Autodesk Inventor part; units mm, degrees
ref_plane "YZ Plane" through (0, 0, 0) normal (1, 0, 0) x (0, 1, 0)
ref_plane "XZ Plane" through (0, 0, 0) normal (0, 1, 0) x (-1, 0, 0)
ref_plane "XY Plane" through (0, 0, 0) normal (0, 0, 1) x (1, 0, 0)
sketch "スケッチ1" plane through (0, 0, 0) normal (0, 0, 1) x (1, 0, 0)
  line L0 (9, 0) -> (9, 4)
  line L1 (9, 12) -> (2.2731, 12)
  line L2 (0, 8) -> (9, 8)
  line L3 (0, 4) -> (9, 4)
  line L4 (9, 8) -> (9, 12)
  line L5 (2.2731, 12) -> (0, 14.2779)
  line L6 (2.2731, 0) -> (-5.7099, -8)
  line L7 (-5.7099, 20) -> (-15.7099, 20)
  line L8 (-5.7099, -8) -> (-15.7099, -8)
  line L9 (-15.7099, 20) -> (-25.7698, 20)
  line L10 (-25.7698, 20) -> (-25.7698, -8)
  line L11 (-25.7698, -8) -> (-15.7099, -8)
  line L12 (2.2731, 0) -> (9, 0)
  line L13 (0, 14.2779) -> (-5.7099, 20)
  arc A0 (-2.1881, 8) -> (-2.1881, 4) centre (-5.7099, 6) ccw
  line L14 (0, 8) -> (-2.1881, 8)
  line L15 (0, 4) -> (-2.1881, 4)
  point P0 (0, 0)
  point P1 (4.5, 12)
  point P2 (4.5, 0)
  point P3 (4.5, 4)
  point P4 (-25.7099, 6)
  dimension "d5" = 4
  dimension "d8" = 10
  dimension "d9" = 10
  dimension "d12" = 14
  dimension "d90" = 8.1
extrude "押し出し1" add sketch "スケッチ1" along normal blind 6
sketch "スケッチ2" plane through (0, 0, 6) normal (0, 0, 1) x (1, 0, 0)
  circle A0 centre (5.6365, 13.3) radius 1.5
  line L0 (9, 8) -> (9, 12)
  line L1 (11.5477, 6) -> (-28.1936, 6) construction
  line L2 (9, 12) -> (2.2731, 12)
  circle A1 centre (5.6365, -1.3) radius 1.5
  point P0 (0, 0)
  point P1 (4.8882, 12)
  point P2 (6.3849, 12)
  dimension "d15" = 3
  dimension "d16" = 3.3635
  dimension "d17" = 1.3
extrude "押し出し2" cut sketch "スケッチ2" against normal blind 6 contours A0 L2 | A1 picked at (5.4614, 13.0013)
sketch "スケッチ3" plane through (0, 0, 6) normal (0, 0, 1) x (1, 0, 0)
  circle A0 centre (5.6365, 13.3) radius 1.5
  line L0 (9, 12) -> (2.2731, 12)
  point P0 (0, 0)
  point P1 (4.8882, 12)
  point P2 (6.3849, 12)
  dimension "d20" = 3
  dimension "d21" = 1.3
extrude "押し出し3" add sketch "スケッチ3" against normal blind 6 contours A0 L0 picked at (5.4614, 13.0013)
sketch "スケッチ4" plane through (0, 0, 6) normal (0, 0, 1) x (1, 0, 0)
  arc A0 (6.3849, 12) -> (4.8882, 12) centre (5.6365, 13.3) ccw
  circle A1 centre (5.6365, 13.3) radius 1.5
  point P0 (0, 0)
  dimension "d24" = 3
extrude "押し出し4" cut sketch "スケッチ4" against normal blind 6
fillet "フィレット1" radius 5 1 edges at (-25.7698, 20, 3)
fillet "フィレット2" radius 5 1 edges at (-25.7698, -8, 3)
fillet "フィレット3" radius 3 4 edges at (-5.7099, -8, 3) (2.2731, 0, 3) (-5.7099, 20, 3) (2.2731, 12, 3)
sketch "スケッチ6" plane through (0, 4, 0) normal (0, 1, 0) x (1, 0, 0)
  point P0 (0, 0)
sketch "スケッチ7" plane through (4.8882, 12, 6) normal (0, 1, 0) x (1, 0, 0)
  circle A0 centre (0.7488, 3) radius 1.6
  line L0 (1.4967, 0) -> (0, 0)
  line L1 (4.1118, 6) -> (4.1118, 0)
  point P0 (-4.8882, 6)
  point P1 (0.7483, 0)
  dimension "d43" = 3.2
  dimension "d44" = 3
  dimension "d45" = 3.363
extrude "押し出し5" cut sketch "スケッチ7" against normal blind 28
sketch "スケッチ11" plane through (0, 0, 6) normal (0, 0, 1) x (1, 0, 0)
  line L0 (-6.9544, 20) -> (-20.7698, 20)
  line L1 (-20.7698, 20) -> (-6.9544, 20)
  arc A0 (1.394, 12.8809) -> (3.5176, 12) centre (3.5176, 15) ccw
  line L2 (0, 20) -> (1.3068, 17.0279)
  arc A1 (1.394, 12.8809) -> (3.5176, 12) centre (3.5176, 15) ccw
  arc A2 (-4.8308, 19.1191) -> (-6.9544, 20) centre (-6.9544, 17) ccw
  arc A3 (-4.8308, 19.1191) -> (-6.9544, 20) centre (-6.9544, 17) ccw
  line L3 (1.394, 12.8809) -> (-4.8308, 19.1191)
  line L4 (-4.8308, 19.1191) -> (1.394, 12.8809)
  arc A4 (0, 8) -> (0, 4) centre (-5.7099, 6) ccw
  line L5 (-11.7599, 6) -> (12.1155, 6) construction
  line L6 (-20.7698, -8) -> (0, -8)
  line L7 (0, -8) -> (3.5176, 0)
  arc A5 (-6.9544, -8) -> (-4.8308, -7.1191) centre (-6.9544, -5) ccw
  line L8 (1.394, -0.8809) -> (-4.8308, -7.1191)
  line L9 (-6.9544, 20) -> (0, 20)
  line L10 (1.3068, 17.0279) -> (3.5176, 12)
  arc A6 (3.5176, 0) -> (1.394, -0.8809) centre (3.5176, -3) ccw
  point P0 (0, 0)
extrude "押し出し6" add sketch "スケッチ11" against normal blind 6
sketch "スケッチ12" plane through (0, 0, 6) normal (0, 0, 1) x (1, 0, 0)
  arc A0 (0, 8) -> (0, 4) centre (-5.7099, 6) ccw
  point P0 (0, 0)
  point P1 (-15.7099, 6)
  point P2 (-5.7099, 16)
  point P3 (-5.7099, -4)
  dimension "d74" = 10
  dimension "d76" = 10
  dimension "d77" = 10
hole "穴4" at (-15.7099, 6, 6) at (-5.7099, 16, 6) at (-5.7099, -4, 6) direction (0, 0, -1) diameter 3.2 end through all
sketch "スケッチ13" plane through (0, 0, 6) normal (0, 0, 1) x (1, 0, 0)
  line L0 (-20.7698, -8) -> (0, -8)
  line L1 (0, 20) -> (-20.7698, 20)
  line L2 (-18.7698, 20) -> (-18.7698, -8) construction
  line L3 (-25.7698, 15) -> (-25.7698, -3)
  arc A0 (-18.7698, 20) -> (-18.7698, -8) centre (6.3784, 6) ccw
  line L4 (-18.7698, 20) -> (-29.3351, 20)
  line L5 (-29.3351, 20) -> (-29.3351, -8)
  line L6 (-29.3351, -8) -> (-18.7698, -8)
  point P0 (0, 0)
  dimension "d85" = 7
extrude "押し出し7" cut sketch "スケッチ13" against normal blind 6
fillet "フィレット4" radius 6 1 edges at (-18.7698, 20, 3)
fillet "フィレット5" radius 6 1 edges at (-18.7698, -8, 3)
properties part number "射出_腕固定2_真" material "ポリカーボネート、クリア"
Read the model definition and answer for the solid it produces. Units are mm, in the model's axes. A direction names the side the tool comes from. Round coordinates to 2 decimals unless told otherwise and drop trailing zeros. Write each loop counter-clockwise with the first axis right and the second up, starting at its lowest first coordinate (ties: lowest second). Pieces come first, ordered by that corner, then holes. Notation, with made-up numbers: (89.5, 50.25) - (136.5, 50.25) arc R31 cw to (136.5, 86.25) - close; hole circle Ø4 at (8, 5.25). An arc over 180 degrees is marked (long way). One line per item, written item: value.
Q1. Find section C-C (z = 3). Determine the outline of the cut face in (x, y), and give its area (3 significant figures).
The answers:
outline: (-20.57, -4.11) arc R6 ccw to (-14.95, -8) - (0, -8) - (3.52, 0) - (4.04, 0) - (4.04, 4) - (-2.19, 4) arc R4.05 cw (long way) to (-2.19, 8) - (4.04, 8) - (4.04, 12) - (3.52, 12) - (1.31, 17.03) - (0, 20) - (-14.95, 20) arc R6 ccw to (-20.57, 16.11) arc R28.78 ccw to start; (7.24, 0) - (9, 0) - (9, 4) - (7.24, 4) - close; (7.24, 8) - (9, 8) - (9, 12) - (7.24, 12) - close; hole circle Ø3.2 at (-15.71, 6); hole circle Ø3.2 at (-5.71, -4); hole circle Ø3.2 at (-5.71, 16)
area: 580 mm2
Q2. For a pull along X with two mould halves and no side action, classify faces 5 (the cylindrical face through (-4.74, 17.27, 2.96)), 6 (the flat face through (-10, 6, 6)), 7 (the flat face through (9, 10, 3)) as pulls with the +X half, pulls with the -X half, needs draft (parallel to the pull), parting line crosses it, or undercut.
The answers:
face 5: undercut
face 6: needs draft
face 7: pulls with the +X half
Q3. Find section D-D (x = 5.5). Determine the outline of the cut face in (y, z), and give its area (3 significant figures).
The answers:
outline: (0.19, 0) - (4, 0) - (4, 1.41) - (0.19, 1.41) - close; (0.19, 4.59) - (4, 4.59) - (4, 6) - (0.19, 6) - close; (8, 0) - (11.81, 0) - (11.81, 1.41) - (8, 1.41) - close; (8, 4.59) - (11.81, 4.59) - (11.81, 6) - (8, 6) - close
area: 21.4 mm2
Q4. Find section A-A (y = 6). Determine the outline of the cut face in (x, z).
The answers:
outline: (-22.4, 0) - (-17.31, 0) - (-17.31, 6) - (-22.4, 6) - close; (-14.11, 0) - (-9.76, 0) - (-9.76, 6) - (-14.11, 6) - close
Q5. Find section B-B (x = -0.5). Determine the outline of the cut face in (y, z).
The answers:
outline: (-8, 0) - (4, 0) - (4, 6) - (-8, 6) - close; (8, 0) - (20, 0) - (20, 6) - (8, 6) - close
Q6. Straight lines are drawn through the part: line 1 (Y direction, x = 6.5, z = 1.25); line 2 (X direction, y = 16.5, z = 5.5); line 3 (Y direction, x = -2.5, z = 5). For each, find the intervals that lie inside material, in ascending order. Write a range as from..to.
The answers:
line 1: y = 0..4, 8..12
line 2: x = -20.41..-7.23, -4.19..1.54
line 3: y = -8..3.53, 8.47..20
Q7. Each of these flat-tipped pins is pushed along its axis until it touches: P1, Ø1.5, axis at x = 4.5, z = 4.5, coming from the +Y side; P2, Ø6.5, axis at x = -5.71, y = 6, coming from the -Z side; P3, Ø2, axis at x = 7.5, z = 3, coming from the -Y side; P4, Ø3, axis at x = 3.5, z = 3, coming from the -Y side. Where does it stop, or does it pass through?
The answers:
P1: stops at y = 12
P2: passes through
P3: stops at y = 0
P4: stops at y = -3.45
Q8. Which of the six approach directions +Z, -Z, +X, -X, +Y, -Y give full straight-line access (tool end or side, diameter ignored) to faces 1 (the cylindrical face through (-4.15, -3.65, 2.96)), 2 (the flat face through (8, 12, 3)), 3 (the flat face through (3, 4, 3)), 4 (the flat face through (3.7, 0, 3))?
The answers:
face 1: +Z, -Z
face 2: +Z, -Z, +X, +Y
face 3: +Z, -Z, +X
face 4: +Z, -Z, +X, -Y
